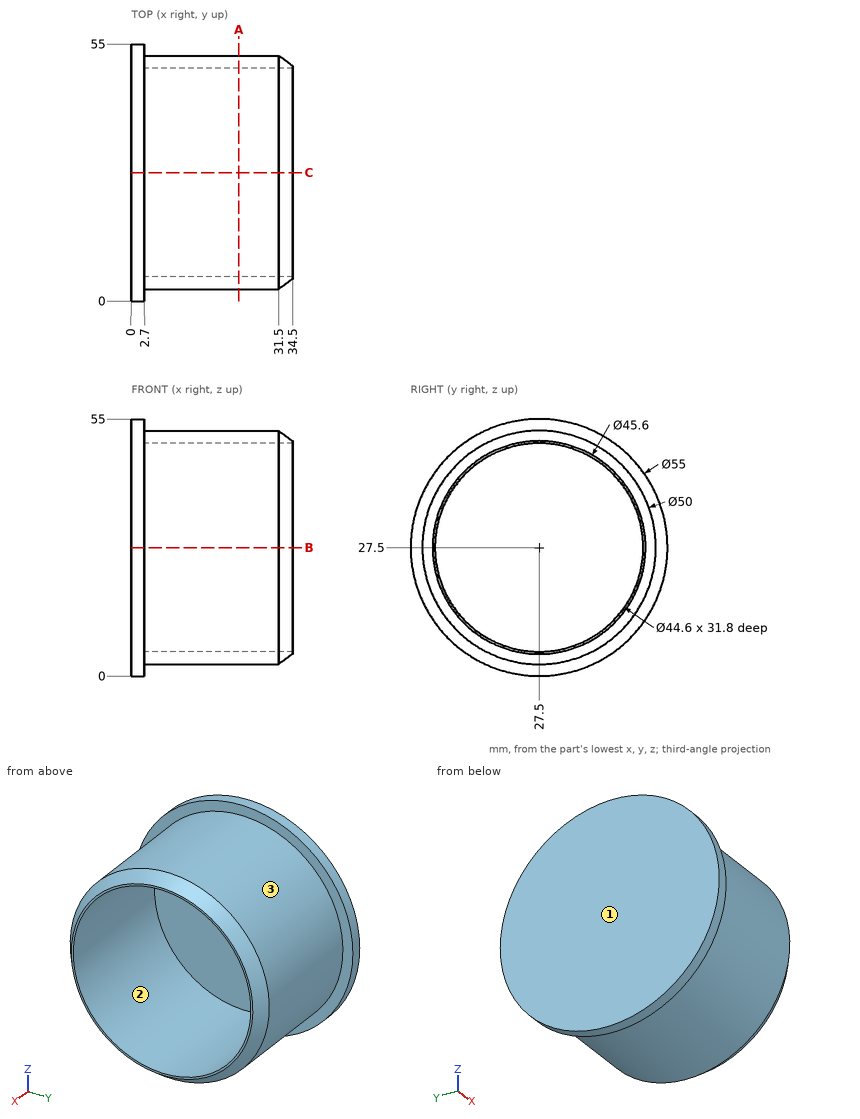
Answer from the drawing. Dimensions are ordinates in mm from the lowest x, y and z of the part. Round coordinates to 2 decimals unless told otherwise and drop trailing zeros. Order: outer loops, then holes, each group sorted by start corner. A loop starts at its lowest first (then second) coordinate and runs counter-clockwise, first axis right, second up.
1) The part is cut by section B-B on z = 27.5. Write down the section's boundary in (x, y).
2) Straight lines are drawn through the part: L1, parallel to Y at x = 17.5, z = 27.5; L2, parallel to X at y = 6, z = 12.5; L3, parallel to Y at x = 22, z = 31.5. For each, find the intervals that lie inside material, in ascending order.
3) The part is cut by section A-A on x = 23. Write down the section's boundary in (y, z), plus the area to 3 significant figures.
4) Flat-ended cylindrical pins translate along their axes: pin 1 (2 mm diameter, centred on y = 28, z = 44.5, fed in from +X); pin 2 (10 mm diameter, centred on x = 19.5, y = 15.5, fed in from +Z); pin 3 (5 mm diameter, centred on x = 28.5, z = 48, fed in from +Y). Find the tip coordinate at first contact, or state that the pin passes through.
5) The mould has two halves that part along Y. Classify the marked faces 1, 2 and 3: released by +Y, released by -Y, zero draft, split by the parting line, or undercut.
Resolved:
1. outline: (0, 0) - (2.7, 0) - (2.7, 2.5) - (31.5, 2.5) - (34.5, 4.7) - (34.5, 5.2) - (2.7, 5.2) - (2.7, 49.8) - (34.5, 49.8) - (34.5, 50.3) - (31.5, 52.5) - (2.7, 52.5) - (2.7, 55) - (0, 55) - close
2. L1: y = 2.5 to 5.2, 49.8 to 52.5
2. L2: x = 0 to 2.7
2. L3: y = 2.82 to 5.56, 49.44 to 52.18
3. outline: circle Ø50 at (27.5, 27.5); hole circle Ø44.6 at (27.5, 27.5)
3. area: 401 mm2
4. pin 1: stops at x = 2.7
4. pin 2: stops at z = 51.5
4. pin 3: stops at y = 44.85
5. face 1: zero draft
5. face 2: undercut
5. face 3: split by the parting line
